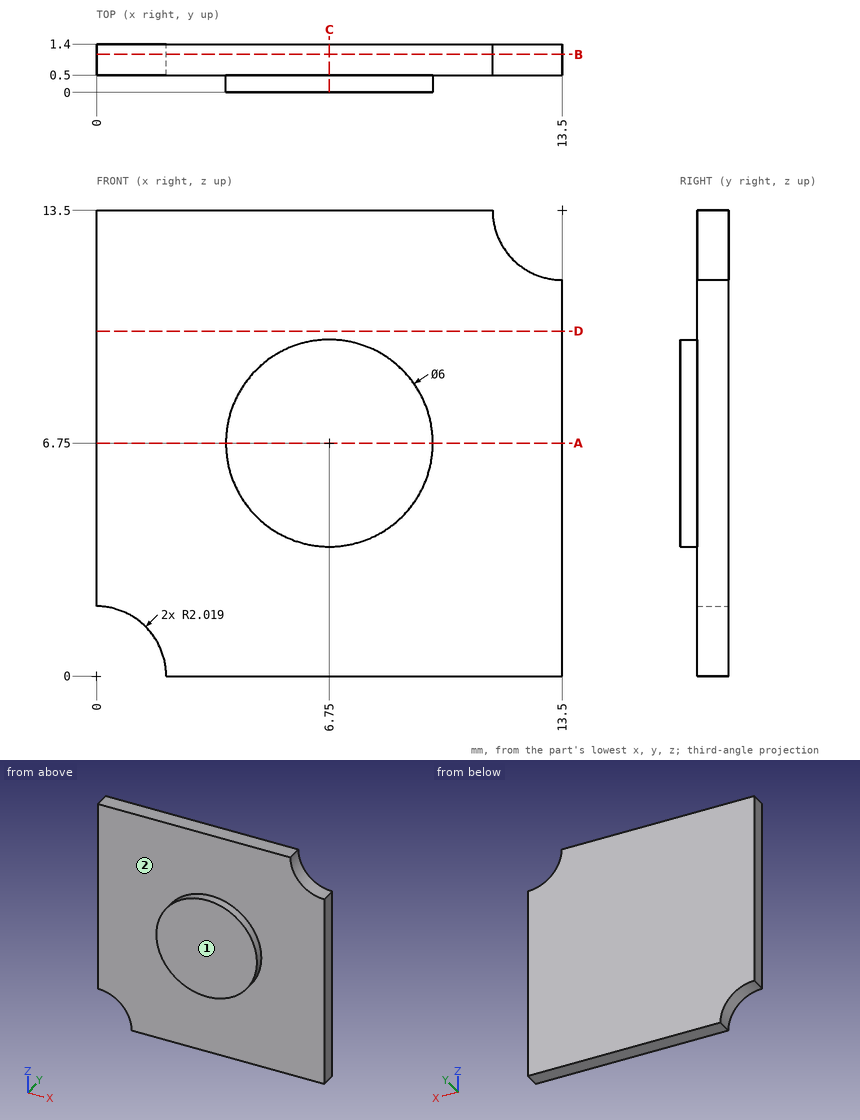
Design review of the part shown in the three views and the two pictorial views. Dimensions are in mm from the part's minimum x, y and z. A direction names the side the tool comes from. Give positions to 0.01 mm unless a question says otherwise; leave off trailing zeros. Loops run counter-clockwise (first coordinate to the right, second up) from the corner with the lowest first, then second, coordinate; pieces in that order, holes last. Notation, with made-up numbers: (4.5, -2.75) -> (54.5, -2.75) arc R23 ccw to (54.5, 20.25) -> close; hole circle Ø5 at (88, -16). An arc over 180 degrees is marked (long way). Answer as a JSON object with one key per item and string values. Group by question number.
Q1. Take a section at D-D (z = 10). Write out the cut boundary in (x, y).
Q2. Take a section at B-B (y = 1.1). Write out the cut boundary in (x, z).
Q3. Take a section at C-C (x = 6.75). Write out the cut boundary in (y, z).
Q4. Tool access review of the marked faces 1 and 2: name each direction out of +Z, -Z, +X, -X, +Y, -Y from which nothing blocks a thin tool from reaching the whole face with its end or side.
Q5. Wall thickness on line 1 along Y through (x, z) = (1.75, 10.5); line 2 along Z through (x, y) = (9.5, 0.25); line 3 along Z through (x, y) = (12.25, 1.15) (1 decimal): over which ranges is each line inside the solid? List them lowest first.
Q6. Take a section at A-A (z = 6.75). Write out the cut boundary in (x, y).
Q7. Insertion check: pin 1 (4 mm diameter, centred on x = 2, z = 6, fed in from -Y). The pin has a flat end and moves straight along its axis. Give the tip position at first contact, or say it passes through.
Answer below:
{
 "1": {"outline": "(0, 0.5) -> (13.5, 0.5) -> (13.5, 1.4) -> (0, 1.4) -> close"},
 "2": {"outline": "(0, 2.02) arc R2.02 cw to (2.02, 0) -> (13.5, 0) -> (13.5, 11.48) arc R2.02 cw to (11.48, 13.5) -> (0, 13.5) -> close"},
 "3": {"outline": "(0, 3.75) -> (0.5, 3.75) -> (0.5, 0) -> (1.4, 0) -> (1.4, 13.5) -> (0.5, 13.5) -> (0.5, 9.75) -> (0, 9.75) -> close"},
 "4": {"face 1": "+Z, -Z, +X, -X, -Y", "face 2": "-Y"},
 "5": {"line 1": "y = 0.5 to 1.4", "line 2": "z = 5.55 to 7.95", "line 3": "z = 0 to 11.9"},
 "6": {"outline": "(0, 0.5) -> (3.75, 0.5) -> (3.75, 0) -> (9.75, 0) -> (9.75, 0.5) -> (13.5, 0.5) -> (13.5, 1.4) -> (0, 1.4) -> close"},
 "7": {"pin 1": "stops at y = 0"}
}
